Geometry: see drawing. Coordinates: mm, zero at the bounding-box minimum. A direction names the side the tool comes from. Give positions to 0.01 mm unless a question says otherwise; leave off trailing zeros. Order: outer loops, then holes, each group sorted by start corner. A loop starts at its lowest first (then second) coordinate and runs counter-clockwise, first axis right, second up. Notation, with made-up numbers: M -18,-21 L -7,-21 A26 ccw -7,12 Z; hole C 7,9 d4. An arc over 180 degrees is marked long. Return JSON: item names as keys, results as strings.
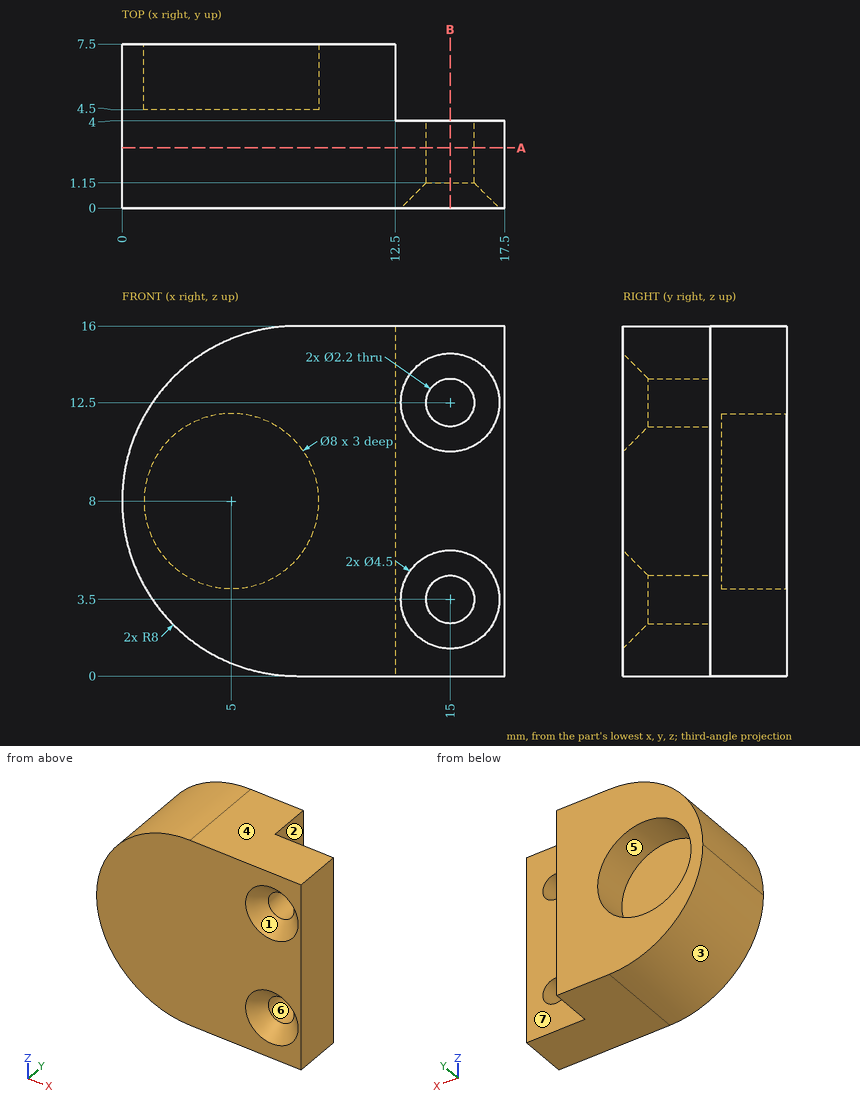
1. Section query A-A (y = 2.75). State how many separate pieces and enclosed holes the cut face has, then the cut area to 3 significant figures.
Evaluation:
{"separate pieces": "1", "enclosed holes": "2", "area": "245 mm^2"}
2. Set-up query: the marked faces 5, 6 and 7. Return all of +Z, -Z, +X, -X, +Y, -Y with unobstructed straight access to the full face (end or side cutting, diameter ignored); none if empty.
Evaluation:
{"face 5": "+Y", "face 6": "+Y, -Y", "face 7": "+Z, -Z, +X, +Y"}
3. First-contact query: pin 1 (4 mm diameter, centred on x = 16, z = 8, fed in from +Y); pin 2 (4 mm diameter, centred on y = 6.5, z = 6, fed in from +X); pin 3 (2 mm diameter, centred on x = 15, z = 3.5, fed in from +Y); pin 4 (2 mm diameter, centred on x = 5.5, y = 4, fed in from +Z). Flat tips, straight axial feed; report the tip coordinate or a pass-through.
Evaluation:
{"pin 1": "stops at y = 4", "pin 2": "stops at x = 12.5", "pin 3": "passes through", "pin 4": "stops at z = 15.86"}
4. Draft query along X for the marked faces 1, 2, 3 and 4. Return one class per face: pulls with the +X half, pulls with the -X half, needs draft (parallel to the pull), parting line crosses it, or undercut.
Evaluation:
{"face 1": "undercut", "face 2": "pulls with the +X half", "face 3": "pulls with the -X half", "face 4": "needs draft"}
5. Section query B-B (x = 15). Return loops of the section in (y, z).
Evaluation:
{"outline": "M 0,0 L 4,0 L 4,2.4 L 1.15,2.4 L 0,1.25 Z; M 0,5.75 L 1.15,4.6 L 4,4.6 L 4,11.4 L 1.15,11.4 L 0,10.25 Z; M 0,14.75 L 1.15,13.6 L 4,13.6 L 4,16 L 0,16 Z"}
6. Ray query, probe 1 along Z at (x, y) = (15, 3.25); probe 2 along Y at (x, z) = (13.75, 6); probe 3 along Z at (x, y) = (5, 6.05) (1 decimal). Return the intervals inside material, ascending.
Evaluation:
{"probe 1": "z = 0 to 2.4, 4.6 to 11.4, 13.6 to 16", "probe 2": "y = 0 to 4", "probe 3": "z = 0.6 to 4, 12 to 15.4"}
